```python
from build123d import *

# Parameters (mm, degrees)
F1_DEPTH    = 228.6
F3_D        = 7.9375
F4_T1_DEPTH = 457.2
F4_T3_DEPTH = 463.55


# Not quite as in the source:
# - a fillet or chamfer that OpenCascade refuses, or shapes differently, is made with other operations: its cross-section is extruded or revolved along the edge and cut away or added


with BuildPart() as f1:
    # F0 (on Front) → F1 (new body, symmetric)
    with BuildSketch(Plane.XZ):
        Polygon((0, 2.264165209), (0, 0), (2.7281190167, 0), (19.05, 0), (19.05, 2.264165209), (2.7281190167, 2.264165209), (2.7281190167, 19.05), (0, 19.05), align=None)
    extrude(amount=F1_DEPTH, both=True)

    # F3 (through all)
    with Locations(Plane.YZ.offset(2.7281190167)):
        with Locations((-203.2, 11.1125), (-152.4, 11.1125), (-101.6, 11.1125), (-50.8, 11.1125), (101.6, 11.1125), (50.8, 11.1125), (0, 11.1125), (152.4, 11.1125), (203.2, 11.1125)):
            Hole(F3_D / 2)

    # F4: fillet of radius 1.27 on 6 edges, made by hand

    # F4_s2 → F4_t1 (join)
    with BuildSketch(Plane.XZ.offset(-228.6)):
        with BuildLine():
            ThreePointArc((3.9981190167, 2.264165209), (3.1000934046, 2.6361395969), (2.7281190167, 3.534165209))
            Line((2.7281190167, 3.534165209), (2.7281190167, 2.264165209))
            Line((2.7281190167, 2.264165209), (3.9981190167, 2.264165209))
        make_face()
    extrude(amount=F4_T1_DEPTH)

    # F4_s4 → F4_t3 (cut)
    with BuildSketch(Plane.XZ.offset(-231.775)):
        with BuildLine():
            ThreePointArc((0, 17.78), (0.3719743879, 18.6780256121), (1.27, 19.05))
            Line((1.27, 19.05), (0, 19.05))
            Line((0, 19.05), (0, 17.78))
        make_face()
        with BuildLine():
            ThreePointArc((1.4581190167, 19.05), (2.3561446288, 18.6780256121), (2.7281190167, 17.78))
            Line((2.7281190167, 17.78), (2.7281190167, 19.05))
            Line((2.7281190167, 19.05), (1.4581190167, 19.05))
        make_face()
        with BuildLine():
            ThreePointArc((19.05, 0.994165209), (18.6780256121, 1.8921908211), (17.78, 2.264165209))
            Line((17.78, 2.264165209), (19.05, 2.264165209))
            Line((19.05, 2.264165209), (19.05, 0.994165209))
        make_face()
        with BuildLine():
            ThreePointArc((17.78, 0), (18.6780256121, 0.3719743879), (19.05, 1.27))
            Line((19.05, 1.27), (19.05, 0))
            Line((19.05, 0), (17.78, 0))
        make_face()
        with BuildLine():
            ThreePointArc((0, 1.27), (0.3719743879, 0.3719743879), (1.27, 0))
            Line((1.27, 0), (0, 0))
            Line((0, 0), (0, 1.27))
        make_face()
    extrude(amount=F4_T3_DEPTH, mode=Mode.SUBTRACT)


solid = f1.part
```
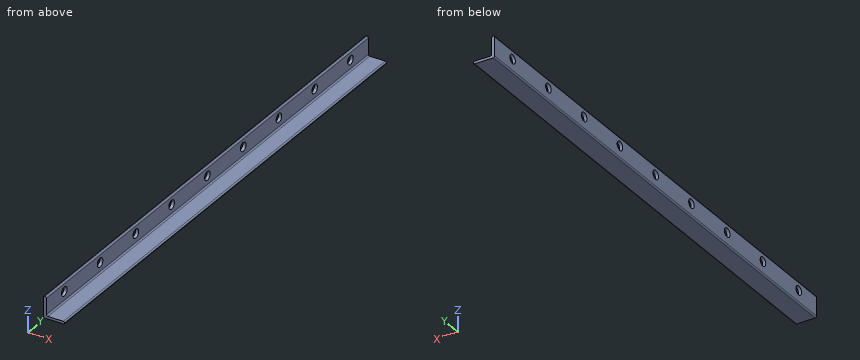
Check sheet for the modelled part. Datum: model origin and axes. Units: mm. Round coordinates to 2 decimals unless told otherwise and drop trailing zeros. Order: outer loops, then holes, each group sorted by start corner. A loop starts at its lowest first (then second) coordinate and runs counter-clockwise, first axis right, second up. Notation, with made-up numbers: (6.5, 42) -> (44.5, 42) arc R27 ccw to (44.5, 77) -> close; hole circle Ø11 at (25.5, 6.25). An arc over 180 degrees is marked (long way). One line per item, written item: value. Start each with the question number.
Q1. Thickness scan on line 1 (Z direction, x = 1.9, y = 50.8); line 2 (Z direction, x = 0.8, y = 203.2); line 3 (X direction, y = 10, z = 1.25). Record the ranges inside material, lowest first.
Q2. Cross-section at A-A (y = 203.2). Record the boundary of the cut face in (x, z), and give its area (3 significant figures).
Q3. Cross-section at B-B (y = -10.5). Record the boundary of the cut face in (x, z), and give its area (3 significant figures).
Q4. Cross-section at C-C (x = 9). Record the boundary of the cut face in (y, z), and give its area (3 significant figures).
Q5. Gauge pin test, flat ends, axial feed: pin 1 Ø4 at (x, y) = (10.5, 157) entering from +Z; pin 2 Ø4.5 at (y, z) = (-99.5, 12.5) entering from +X; pin 3 Ø8 at (y, z) = (34, 5.5) entering from +X. Record the tip position at first contact, or that the pin passes through.
Completed:
1. line 1: z = 0 to 7.14, 15.08 to 18.97
1. line 2: z = 0.09 to 7.14, 15.08 to 18.96
1. line 3: x = 0 to 19.02
2. outline: (0, 1.27) arc R1.27 ccw to (1.27, 0) -> (17.78, 0) arc R1.27 ccw to (19.04, 1.13) arc R1.27 ccw to (17.78, 2.26) -> (4, 2.26) arc R1.27 cw to (2.73, 3.53) -> (2.73, 7.14) -> (0, 7.14) -> close; (0, 15.08) -> (2.73, 15.08) -> (2.73, 17.78) arc R1.27 ccw to (1.46, 19.05) -> (1.27, 19.05) arc R1.27 ccw to (0, 17.78) -> close
2. area: 65.9 mm²
3. outline: (0, 1.27) arc R1.27 ccw to (1.27, 0) -> (17.78, 0) arc R1.27 ccw to (19.04, 1.13) arc R1.27 ccw to (17.78, 2.26) -> (4, 2.26) arc R1.27 cw to (2.73, 3.53) -> (2.73, 17.78) arc R1.27 ccw to (1.46, 19.05) -> (1.27, 19.05) arc R1.27 ccw to (0, 17.78) -> close
3. area: 87.5 mm²
4. outline: (-228.6, 0) -> (228.6, 0) -> (228.6, 2.26) -> (-228.6, 2.26) -> close
4. area: 1,040 mm²
5. pin 1: stops at z = 2.26
5. pin 2: stops at x = 2.73
5. pin 3: stops at x = 18.94
